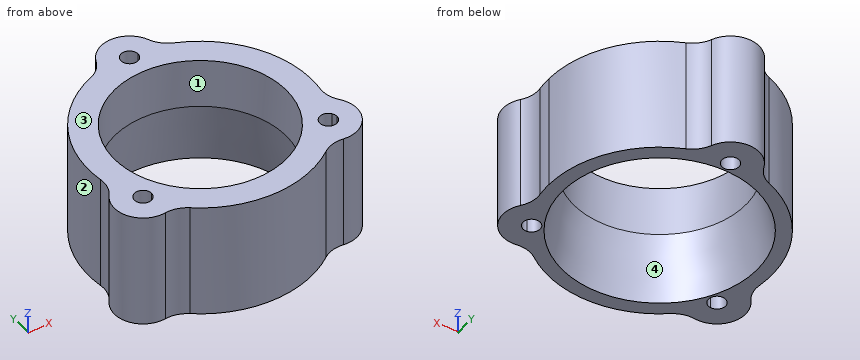
from build123d import *

# Parameters (mm, degrees)
F0_R     = 19.05
F1_DEPTH = 25.4
F2_R     = 6.35
F3_SIZE2 = 14.4050558218
F3_SIZE  = 2.54


with BuildPart() as f1:
    # F0 (on Top) → F1 (new body)
    with BuildSketch(Plane.XY):
        with BuildLine():
            ThreePointArc((23.7041161885, -4.5293078328), (24.3480999851, -1.3231236326), (24.564016243, 1.9399596371))
            ThreePointArc((24.564016243, 1.9399596371), (19.4276047684, 17.0404145143), (6.149016243, 25.8770172048))
            ThreePointArc((6.149016243, 25.8770172048), (3.8641251316, 26.3690430158), (1.5430253852, 26.6434747131))
            ThreePointArc((1.5430253852, 26.6434747131), (1.6633341365, 26.2686085633), (1.704016243, 25.8770172048))
            ThreePointArc((1.704016243, 25.8770172048), (-0.5925751155, 24.0126993113), (-1.9449928991, 26.6434747131))
            ThreePointArc((-1.9449928991, 26.6434747131), (-4.2660926456, 26.3690430158), (-6.550983757, 25.8770172048))
            ThreePointArc((-6.550983757, 25.8770172048), (-21.6481028817, 14.3224596371), (-24.1060837025, -4.5293078328))
            ThreePointArc((-24.1060837025, -4.5293078328), (-23.3897449984, -6.7540944856), (-22.4668599467, -8.9014416794))
            ThreePointArc((-22.4668599467, -8.9014416794), (-20.3380528201, -8.218226811), (-19.0260837025, -10.0285691468))
            ThreePointArc((-19.0260837025, -10.0285691468), (-19.5123327253, -11.2998561579), (-20.7228508045, -11.9221541225))
            ThreePointArc((-20.7228508045, -11.9221541225), (-19.3246361098, -13.795069619), (-17.7560837025, -15.5278304608))
            ThreePointArc((-17.7560837025, -15.5278304608), (-0.200983757, -22.8250403629), (17.3541161885, -15.5278304608))
            ThreePointArc((17.3541161885, -15.5278304608), (18.9226685958, -13.795069619), (20.3208832906, -11.9221541225))
            ThreePointArc((20.3208832906, -11.9221541225), (18.8793377943, -9.0760691468), (22.0648924327, -8.9014416794))
            ThreePointArc((22.0648924327, -8.9014416794), (22.9877774845, -6.7540944856), (23.7041161885, -4.5293078328))
        make_face()
        with Locations((-0.200983757, 1.9399596371)):
            Circle(F0_R, mode=Mode.SUBTRACT)
        with BuildLine():
            ThreePointArc((1.5430253852, 26.6434747131), (3.8641251316, 26.3690430158), (6.149016243, 25.8770172048))
            ThreePointArc((6.149016243, 25.8770172048), (-0.200983757, 32.2270172048), (-6.550983757, 25.8770172048))
            ThreePointArc((-6.550983757, 25.8770172048), (-4.2660926456, 26.3690430158), (-1.9449928991, 26.6434747131))
            ThreePointArc((-1.9449928991, 26.6434747131), (-0.200983757, 27.7820172048), (1.5430253852, 26.6434747131))
        make_face()
        with BuildLine():
            ThreePointArc((17.3541161885, -15.5278304608), (26.0283775025, -13.2035691468), (23.7041161885, -4.5293078328))
            ThreePointArc((23.7041161885, -4.5293078328), (22.9877774845, -6.7540944856), (22.0648924327, -8.9014416794))
            ThreePointArc((22.0648924327, -8.9014416794), (22.3394585243, -9.4355382645), (22.4341161885, -10.0285691468))
            ThreePointArc((22.4341161885, -10.0285691468), (21.8004031997, -11.447320124), (20.3208832906, -11.9221541225))
            ThreePointArc((20.3208832906, -11.9221541225), (18.9226685958, -13.795069619), (17.3541161885, -15.5278304608))
        make_face()
        with BuildLine():
            ThreePointArc((-22.4668599467, -8.9014416794), (-23.3897449984, -6.7540944856), (-24.1060837025, -4.5293078328))
            ThreePointArc((-24.1060837025, -4.5293078328), (-26.4303450165, -13.2035691468), (-17.7560837025, -15.5278304608))
            ThreePointArc((-17.7560837025, -15.5278304608), (-19.3246361098, -13.795069619), (-20.7228508045, -11.9221541225))
            ThreePointArc((-20.7228508045, -11.9221541225), (-22.5808620967, -10.9810691468), (-22.4668599467, -8.9014416794))
        make_face()
    extrude(amount=F1_DEPTH)

    # F2
    f2_edges = [f1.edges().sort_by_distance(p)[0] for p in [
        (-24.106084, -4.529308, 12.7),
        (17.354116, -15.52783, 12.7),
        (6.149016, 25.877017, 12.7),
        (23.704116, -4.529308, 12.7),
        (-6.550984, 25.877017, 12.7),
        (-17.756084, -15.52783, 12.7),
    ]]
    fillet(f2_edges, radius=F2_R)

    # F3
    f3_edges = [f1.edges().sort_by_distance(p)[0] for p in [
        (-19.250984, 1.93996, 0),
    ]]
    f3_side = f1.faces().sort_by_distance((20.577327, 13.936323, 0))[0]
    chamfer(f3_edges, length=F3_SIZE, length2=F3_SIZE2, reference=f3_side)


solid = f1.part
Check sheet for the modelled part. Datum: model origin and axes. Units: mm. Face numbers are marked on the shaded views. Round coordinates to 2 decimals unless told otherwise and drop trailing zeros. One line per item, written item: value. Start each with the question number.
1. Section check A-A on z = 9. Give the number of separate pieces and of enclosed holes in the cut face, and give its area (3 significant figures).
2. Gauge pin test, flat ends, axial feed: P1, Ø1.5, axis at x = -18, z = 6, coming from the +Y side; P2, Ø2, axis at x = -14.5, z = 13, coming from the -Y side; P3, Ø4, axis at y = 3, z = 7.5, coming from the +X side. Record the tip position at first contact, or that the pin passes through.
3. Scan lines: line 1 along Y through (x, z) = (1, 6.25); line 2 along Y through (x, z) = (19, 3.5); line 3 along Y through (x, z) = (11.5, 13). Record each from-to range of solid material in increasing order.
4. Release check for a two-part mould opening along X. For the marked faces 1, 2, 3 and 4 record: released by +X, released by -X, zero draft, split by the parting line, or undercut.
Results found:
1. separate pieces: 1
1. enclosed holes: 4
1. area: 813 mm^2
2. P1: y = 19.9
2. P2: y = -18.95
2. P3: x = 24.56
3. line 1: -22.8 to -18.51, 22.39 to 24.4, 27.36 to 32.11
3. line 2: -16.27 to -11.16, -8.89 to -6.5, 10.38 to 17.58
3. line 3: -19.89 to -13.41, 17.29 to 23.77
4. face 1: undercut
4. face 2: released by -X
4. face 3: zero draft
4. face 4: undercut
